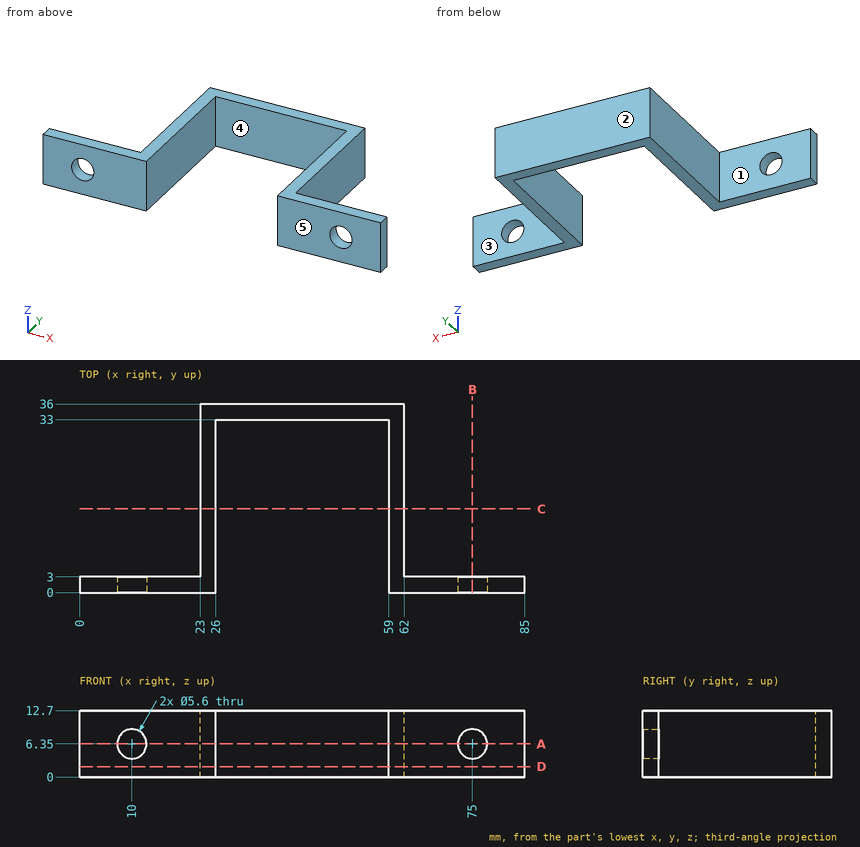
For this review, use the dimensioned drawing (mm, ordinates from the lowest corner) and the shaded views. A direction names the side the tool comes from. Give positions to 0.01 mm unless a question says otherwise; leave off trailing zeros. Order: outer loops, then holes, each group sorted by start corner. A loop starts at its lowest first (then second) coordinate and runs counter-clockwise, first axis right, second up.
1) Wall thickness on line 1 (X direction, y = 0.85, z = 6.35); line 2 (Z direction, x = 75, y = 0.9); line 3 (X direction, y = 30, z = 10.25): over which ranges is each line inside the solid? List them lowest first.
2) Take a section at D-D (z = 2). Give the boundary of the cut face in (x, y), then the cut area to 3 significant figures.
3) Insertion check: pin 1 (4 mm diameter, centred on y = 10.5, z = 6, fed in from +X); pin 2 (5 mm diameter, centred on x = 69, z = 2, fed in from +Y); pin 3 (4 mm diameter, centred on y = 22, z = 4.5, fed in from -X). Each pin has a flat end and moves straight along its axis. Give the tip position at first contact, or say it passes through.
4) Take a section at B-B (x = 75). Give the boundary of the cut face in (y, z), then the cut area to 3 significant figures.
5) Take a section at A-A (z = 6.35). Give the boundary of the cut face in (x, y), then the cut area to 3 significant figures.
6) Take a section at C-C (y = 16). Give the boundary of the cut face in (x, z), then the cut area to 3 significant figures.
7) For the marked faces 1, 2, 3, 4 and 5, list the 3-axis set-ups (+Z, -Z, +X, -X, +Y, -Y) from which the entire face can be reached by the end or side of a thin tool; tool diameter is ignored.
Derived:
1. line 1: x = 0 to 7.2, 12.8 to 26, 59 to 72.2, 77.8 to 85
1. line 2: z = 0 to 3.55, 9.15 to 12.7
1. line 3: x = 23 to 26, 59 to 62
2. outline: (0, 0) - (26, 0) - (26, 33) - (59, 33) - (59, 0) - (85, 0) - (85, 3) - (62, 3) - (62, 36) - (23, 36) - (23, 3) - (0, 3) - close
2. area: 453 mm2
3. pin 1: stops at x = 62
3. pin 2: stops at y = 3
3. pin 3: stops at x = 23
4. outline: (0, 0) - (3, 0) - (3, 3.55) - (0, 3.55) - close; (0, 9.15) - (3, 9.15) - (3, 12.7) - (0, 12.7) - close
4. area: 21.3 mm2
5. outline: (0, 0) - (7.2, 0) - (7.2, 3) - (0, 3) - close; (12.8, 0) - (26, 0) - (26, 33) - (59, 33) - (59, 0) - (72.2, 0) - (72.2, 3) - (62, 3) - (62, 36) - (23, 36) - (23, 3) - (12.8, 3) - close; (77.8, 0) - (85, 0) - (85, 3) - (77.8, 3) - close
5. area: 419 mm2
6. outline: (23, 0) - (26, 0) - (26, 12.7) - (23, 12.7) - close; (59, 0) - (62, 0) - (62, 12.7) - (59, 12.7) - close
6. area: 76.2 mm2
7. face 1: +Z, -Z, -X, +Y
7. face 2: +Z, -Z, +X, -X, +Y
7. face 3: +Z, -Z, +X, +Y
7. face 4: +Z, -Z, -Y
7. face 5: +Z, -Z, +X, -X, -Y
